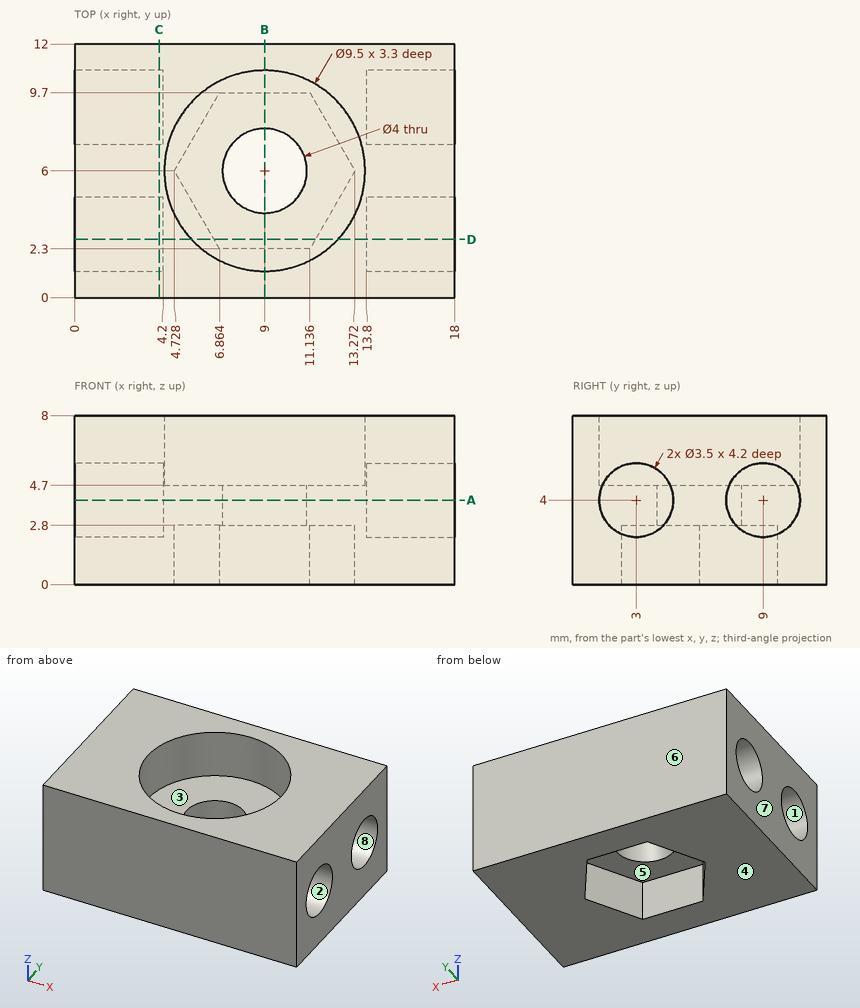
Could you check a few things on this drawing? It's one solid part, dimensions in mm from its lowest x, y, z. A direction names the side the tool comes from. Round coordinates to 2 decimals unless told otherwise and drop trailing zeros. Loops run counter-clockwise (first coordinate to the right, second up) from the corner with the lowest first, then second, coordinate; pieces in that order, holes last.
Q1. For P1, Ø5, axis at x = 7, y = 6, coming from the +Z side; P2, Ø1.8, axis at y = 9.5, z = 3.5, coming from the +X side; P3, Ø1, axis at y = 8.5, z = 4.5, coming from the -X side, each with a flat end and sliding along its axis, tell me the tip position at first contact or that it passes through.
Q2. On a 3-axis mill with a long thin cutter (end or side, diameter ignored), from which of +Z, -Z, +X, -X, +Y, -Y can I reach the whole of each face in a straight line? I mean the marked faces 1, 2, 3, 4 and 5. Say none if no direction works.
Q3. I want a section at D-D (y = 2.75). Write out the boundary of the cut face in (x, z).
Q4. Please list where these lines run through material, in increasing order: L1, parallel to X at y = 6, z = 6.85; L2, parallel to Z at x = 16.15, y = 3; L3, parallel to Y at x = 8, z = 1.
Q5. I want a section at B-B (x = 9). Write out the boundary of the cut face in (y, z).
Q6. I want a section at A-A (z = 4). Write out the boundary of the cut face in (x, y).
Q7. I want a section at C-C (x = 4). Write out the boundary of the cut face in (y, z).
Q8. Thinking about a two-plate mould opening in Y: for the marked faces 6, 7 and 8, which applies, pulls with the +Y half, pulls with the -Y half, needs draft (parallel to the pull), parting line crosses it, or undercut?
Answer below:
1. P1: stops at z = 4.7
1. P2: stops at x = 13.8
1. P3: stops at x = 4.2
2. face 1: -X
2. face 2: +X
2. face 3: +Z
2. face 4: -Z, +X, -X, +Y, -Y
2. face 5: -Z
3. outline: (0, 0) - (6.6, 0) - (6.6, 2.8) - (11.4, 2.8) - (11.4, 0) - (18, 0) - (18, 2.27) - (13.8, 2.27) - (13.8, 5.73) - (18, 5.73) - (18, 8) - (12.46, 8) - (12.46, 4.7) - (5.54, 4.7) - (5.54, 8) - (0, 8) - (0, 5.73) - (4.2, 5.73) - (4.2, 2.27) - (0, 2.27) - close
4. L1: x = 0 to 4.25, 13.75 to 18
4. L2: z = 0 to 2.25, 5.75 to 8
4. L3: y = 0 to 2.3, 9.7 to 12
5. outline: (0, 0) - (2.3, 0) - (2.3, 2.8) - (4, 2.8) - (4, 4.7) - (1.25, 4.7) - (1.25, 8) - (0, 8) - close; (8, 2.8) - (9.7, 2.8) - (9.7, 0) - (12, 0) - (12, 8) - (10.75, 8) - (10.75, 4.7) - (8, 4.7) - close
6. outline: (0, 0) - (18, 0) - (18, 1.25) - (13.8, 1.25) - (13.8, 4.75) - (18, 4.75) - (18, 7.25) - (13.8, 7.25) - (13.8, 10.75) - (18, 10.75) - (18, 12) - (0, 12) - (0, 10.75) - (4.2, 10.75) - (4.2, 7.25) - (0, 7.25) - (0, 4.75) - (4.2, 4.75) - (4.2, 1.25) - (0, 1.25) - close; hole circle Ø4 at (9, 6)
7. outline: (0, 0) - (12, 0) - (12, 8) - (0, 8) - close; hole circle Ø3.5 at (3, 4); hole circle Ø3.5 at (9, 4)
8. face 6: pulls with the +Y half
8. face 7: needs draft
8. face 8: undercut
